Design review of the part built by this model. Coordinates are the model's own, in mm. A direction names the side the tool comes from. Coordinates: 2 decimals unless noted, no trailing zeros. Loops run counter-clockwise (first coordinate to the right, second up) from the corner with the lowest first, then second, coordinate; pieces in that order, holes last.
Solid Edge part; units mm, degrees
sketch "Sketch1" plane through (0, 0, 0) normal (0, 0, 1) x (1, 0, 0)
  circle A0 centre (0, 0) radius 25
extrude "Protrusion1" add sketch "Sketch1" along normal blind 10
sketch "Sketch2" plane through (0, 0, 10) normal (0, 0, 1) x (1, 0, 0)
  circle A0 centre (0, 0) radius 15
extrude "ExtrudedProtrusion_2" add sketch "Sketch2" along normal blind 20
sketch "Sketch3" plane through (0, 0, 30) normal (0, 0, 1) x (1, 0, 0)
  circle A0 centre (0, 0) radius 10
extrude "ExtrudedCutout_1" cut sketch "Sketch3" against normal blind 10
cosmetic_thread "Thread1"
Q1. Take a section at B-B, the plane z = 24.5. Write out the cut boundary in (x, y), then the cut area to 3 significant figures.
Q2. The part is to be moulded in two halves that separate along Y. For faces 3 (the flat face through (0, 0, 20)), 4 (the cylindrical face through (23.846, -7.509, 4.93)), 5 (the flat face through (0, 0, 0)), say which applies: pulls with the +Y half, pulls with the -Y half, needs draft (parallel to the pull), parting line crosses it, or undercut.
Q3. Take a section at D-D, the plane z = 19. Write out the cut boundary in (x, y).
Q4. Machinability: for faces 1 (the flat face through (3, -10, 30)), 2 (the flat face through (11, -11, 10)), which of the approach directions +Z, -Z, +X, -X, +Y, -Y give a long, thin tool a straight path to every point of the face, cutting with its end or side? Answer none if there is none.
Q5. For line 1 (Y direction, x = 0, z = 22); line 2 (X direction, y = 1.5, z = 23); line 3 (Y direction, x = 9, z = 22.25), list the stretches that pass through material, from the lowest coordinate up.
Q6. Clearance check with flat-ended pins moving along their axes: pin 1 Ø12 at (x, z) = (-11, 6) entering from -Y; pin 2 Ø1.5 at (x, z) = (8, 5.5) entering from -Y; pin 3 Ø3 at (x, z) = (-0.5, 18.5) entering from -Y. State where each tip first meets the part, or that it passes through.
Q7. Take a section at A-A, the plane x = 0. Write out the cut boundary in (y, z), then the cut area to 3 significant figures.
Entries:
1. outline: circle Ø30 at (0, 0); hole circle Ø20 at (0, 0)
1. area: 393 mm2
2. face 3: undercut
2. face 4: parting line crosses it
2. face 5: needs draft
3. outline: circle Ø30 at (0, 0)
4. face 1: +Z, +X, -X, +Y, -Y
4. face 2: +Z
5. line 1: y = -15 to -10, 10 to 15
5. line 2: x = -14.92 to -9.89, 9.89 to 14.92
5. line 3: y = -12 to -4.36, 4.36 to 12
6. pin 1: stops at y = -24.49
6. pin 2: stops at y = -23.93
6. pin 3: stops at y = -15
7. outline: (-25, 0) - (25, 0) - (25, 10) - (15, 10) - (15, 30) - (10, 30) - (10, 20) - (-10, 20) - (-10, 30) - (-15, 30) - (-15, 10) - (-25, 10) - close
7. area: 900 mm2
